The listing builds one solid part. Answer for the finished solid, in the listing's coordinates (mm). Face numbers are marked on the shaded views. A direction names the side the tool comes from. Round coordinates to 2 decimals unless told otherwise and drop trailing zeros. Order: outer loops, then holes, each group sorted by start corner. A loop starts at its lowest first (then second) coordinate and runs counter-clockwise, first axis right, second up. Notation, with made-up numbers: (81, -21.75) -> (112, -21.75) arc R24 cw to (112, 0.25) -> close; hole circle Ø4 at (70.25, 33.5). An arc over 180 degrees is marked (long way). Return JSON: item names as keys, results as strings. Group by question number.
(1) Consider line 1 (Y direction, x = 2.5, z = 9); line 2 (X direction, y = 65.5, z = 9.75); line 3 (Y direction, x = 0, z = 1.95). Determine where each line is inside the solid, lowest interval first. Write a range as [from, to].
(2) Determine the mould class of the marked faces 4, 5, 6 and 7 for opening direction X: +X half, -X half, draft (parallel to the pull), parting line (faces both ways), or undercut.
(3) Which of the six approach directions +Z, -Z, +X, -X, +Y, -Y give full straight-line access (tool end or side, diameter ignored) to the marked faces 1, 2 and 3?
(4) The part is cut by section C-C (x = -60). Determine the outline of the cut face in (y, z), plus the area to 3 significant figures.
(5) The part is cut by section B-B (z = 9.25). Count the separate pieces of the cut face and the enclosed holes in it, plus the area to 3 significant figures.
(6) The part is cut by section A-A (x = 0). Determine the outline of the cut face in (y, z), plus the area to 3 significant figures.
(7) Each of these flat-tipped pins is pushed along its axis until it touches: pin 1 (4 mm diameter, centred on y = 58, z = 15, fed in from +X); pin 2 (6 mm diameter, centred on y = -6, z = 3, fed in from -X); pin 3 (5 mm diameter, centred on x = 30, y = 51.96, fed in from +Z); pin 4 (4 mm diameter, centred on x = -40, z = 10, fed in from +Y). Where does it stop, or does it pass through?
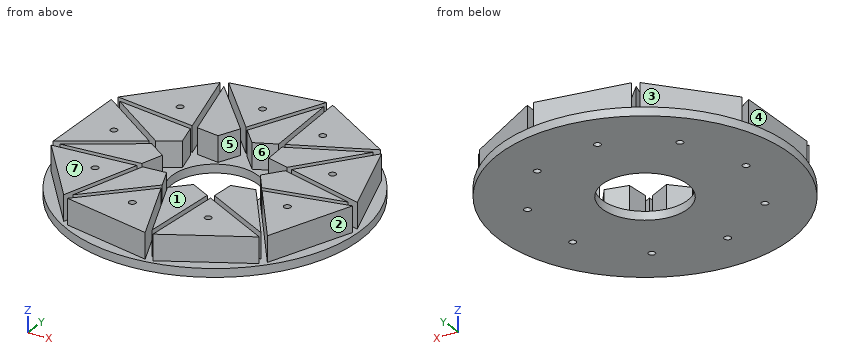
from build123d import *

# Parameters (mm, degrees)
SKETCH002_R   = 85.5
SKETCH002_R_2 = 25
PAD_DEPTH     = 5
PAD001_DEPTH  = 20
SKETCH001_R   = 2
POCKET_DEPTH  = 20.001


with BuildPart() as part:
    # Sketch002 → Pad (new body)
    with BuildSketch(Plane.XY):
        Circle(SKETCH002_R)
        Circle(SKETCH002_R_2, mode=Mode.SUBTRACT)
    extrude(amount=PAD_DEPTH)

    # Sketch → Pad001 (join)
    with BuildSketch(Plane.XY):
        Polygon((16.521561, 81.502157), (62.322158, 55.05917), (19.550743, 33.86288), align=None)
        Polygon((-39.732327, 73.054129), (12.350191, 82.237682), (-6.789902, 38.507446), align=None)
        Polygon((13.742249, 77.936164), (-4.545372, 36.15361), (4.670681, 26.488746), (16.636515, 32.418672), align=None)
        Polygon((19.757136, 30.616981), (60.623574, 50.869218), (33.582631, 14.140398), (20.604587, 17.289301), align=None)
        Polygon((65.044827, 51.81442), (36.743377, 13.373496), (83.132895, 2.11786), align=None)
        Polygon((34.81506, 10.754326), (79.138455, 0), (34.81506, -10.754326), (26.897378, 0), align=None)
        Polygon((36.743377, -13.373496), (83.132895, -2.11786), (65.044827, -51.81442), align=None)
        Polygon((20.604587, -17.289301), (33.582631, -14.140398), (60.623574, -50.869218), (19.757136, -30.616981), align=None)
        Polygon((19.550743, -33.86288), (16.521561, -81.502157), (62.322158, -55.05917), align=None)
        Polygon((4.670681, -26.488746), (16.636515, -32.418672), (13.742249, -77.936164), (-4.545372, -36.15361), align=None)
        Polygon((-6.789902, -38.507446), (12.350191, -82.237682), (-39.732327, -73.054129), align=None)
        Polygon((-26.721049, -24.773563), (-13.448689, -23.293813), (-8.094011, -35.527889), (-39.569228, -68.535913), align=None)
        Polygon((-29.953476, -25.13395), (-43.400568, -70.936269), (-77.395018, -30.423262), align=None)
        Polygon((-74.365822, -27.066946), (-36.393651, -1.801691), (-25.275268, -9.199445), (-29.037259, -22.013212), align=None)
        Polygon((-39.101485, 0), (-78.843719, -26.442988), (-78.843719, 26.442988), align=None)
        Polygon((-74.365822, 27.066946), (-36.393651, 1.801691), (-25.275268, 9.199445), (-29.037259, 22.013212), align=None)
        Polygon((-77.395018, 30.423262), (-43.400568, 70.936269), (-29.953476, 25.13395), align=None)
        Polygon((-39.569228, 68.535913), (-26.721049, 24.773563), (-13.448689, 23.293813), (-8.094011, 35.527889), align=None)
    extrude(amount=PAD001_DEPTH)

    # Sketch001 → Pocket (cut, through all)
    with BuildSketch(Plane.XY):
        with Locations((-10.418201, 59.088587)):
            Circle(SKETCH001_R)
        with Locations((30.000606, 51.961174)):
            Circle(SKETCH001_R)
        with Locations((-45.962216, 38.567793)):
            Circle(SKETCH001_R)
        with Locations((-60, 0.0007)):
            Circle(SKETCH001_R)
        with Locations((-45.963117, -38.56672)):
            Circle(SKETCH001_R)
        with Locations((-10.41958, -59.088344)):
            Circle(SKETCH001_R)
        with Locations((29.999394, -51.961874)):
            Circle(SKETCH001_R)
        with Locations((56.381318, -20.521867)):
            Circle(SKETCH001_R)
        with Locations((56.381797, 20.520551)):
            Circle(SKETCH001_R)
    extrude(amount=POCKET_DEPTH, mode=Mode.SUBTRACT)


solid = part.part
Answer below:
{
 "1": {"line 1": "y = [-80.5, -59.73], [-52.25, -28.77], [28.77, 52.25], [59.73, 80.5]", "line 2": "x = [-47.96, -41.8], [-38.68, -36.67], [-32.53, 5.02], [8.3, 14.53], [17.54, 44.24]", "line 3": "y = [-85.5, -25], [25, 85.5]"},
 "2": {"face 4": "-X half", "face 5": "undercut", "face 6": "undercut", "face 7": "draft"},
 "3": {"face 1": "+Z, +X, -X, +Y, -Y", "face 2": "+Z, +X, -Y", "face 3": "+Z, -X, +Y"},
 "4": {"outline": "(-60.91, 0) -> (-2, 0) -> (-2, 20) -> (-13.91, 20) -> (-13.91, 5) -> (-17.51, 5) -> (-17.51, 20) -> (-25.47, 20) -> (-25.47, 5) -> (-28.48, 5) -> (-28.48, 20) -> (-51.15, 20) -> (-51.15, 5) -> (-60.91, 5) -> close; (2, 0) -> (60.91, 0) -> (60.91, 5) -> (51.15, 5) -> (51.15, 20) -> (28.48, 20) -> (28.48, 5) -> (25.47, 5) -> (25.47, 20) -> (17.51, 20) -> (17.51, 5) -> (13.91, 5) -> (13.91, 20) -> (2, 20) -> close", "area": "1,870 mm²"},
 "5": {"separate pieces": "18", "enclosed holes": "9", "area": "14,400 mm²"},
 "6": {"outline": "(-85.5, 0) -> (-25, 0) -> (-25, 5) -> (-31.39, 5) -> (-31.39, 20) -> (-46.54, 20) -> (-46.54, 5) -> (-54.02, 5) -> (-54.02, 20) -> (-80.06, 20) -> (-80.06, 5) -> (-85.5, 5) -> close; (25, 0) -> (85.5, 0) -> (85.5, 5) -> (80.06, 5) -> (80.06, 20) -> (54.02, 20) -> (54.02, 5) -> (46.54, 5) -> (46.54, 20) -> (31.39, 20) -> (31.39, 5) -> (25, 5) -> close", "area": "1,840 mm²"},
 "7": {"pin 1": "stops at x = 60.69", "pin 2": "stops at x = -85.45", "pin 3": "stops at z = 20", "pin 4": "stops at y = 73.36"}
}
